The model under review builds one solid part; all positions refer to its coordinate system, in mm. Face numbers are marked on the shaded views. A direction names the side the tool comes from. Coordinates: 2 decimals unless noted, no trailing zeros. Write each loop counter-clockwise with the first axis right and the second up, starting at its lowest first coordinate (ties: lowest second). Pieces come first, ordered by that corner, then holes.
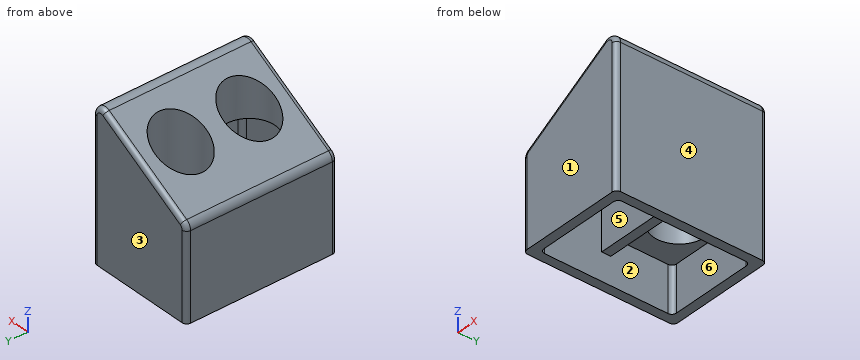
Autodesk Inventor part; units mm, degrees
ref_plane "YZ Plane" through (0, 0, 0) normal (1, 0, 0) x (0, 1, 0)
ref_plane "XZ Plane" through (0, 0, 0) normal (0, 1, 0) x (-1, 0, 0)
ref_plane "XY Plane" through (0, 0, 0) normal (0, 0, 1) x (1, 0, 0)
sketch "Sketch1" plane through (0, 0, 0) normal (0, 1, 0) x (-1, 0, 0)
  line L0 (0, 0) -> (12, 0)
  line L1 (12, 0) -> (12, -10)
  line L2 (12, -10) -> (0, -10)
  line L3 (0, -10) -> (0, 0)
  line L4 (12, 0) -> (0, 6.9282)
  line L5 (12, 0) -> (25.8564, 0) construction
  line L6 (0, 6.9282) -> (0, 0)
  dimension "d0" = 10
  dimension "d1" = 12
  dimension "d2" = 150
extrude "Extrusion1" add sketch "Sketch1" along normal blind 16.5
sketch "Sketch2" plane through (0, 0, -10) normal (0, 0, -1) x (-1, 0, 0)
  circle A0 centre (6, 4.5) radius 2.8
  circle A1 centre (6, 12) radius 2.8
  line L0 (0, 0) -> (0, 16.5)
  line L1 (0, 0) -> (12, 0)
  line L2 (0, 16.5) -> (12, 16.5)
  dimension "d5" = 5.6
  dimension "d6" = 6
  dimension "d7" = 4.5
  dimension "d8" = 4.5
extrude "Extrusion2" cut sketch "Sketch2" against normal through all
fillet "Fillet1" radius 1 2 edges at (0, 8.25, 6.9282) (-12, 8.25, 0)
sketch "Sketch3" plane through (0, 0, -10) normal (0, 0, -1) x (-1, 0, 0)
  circle A0 centre (6, 12) radius 2.8
  circle A1 centre (6, 4.5) radius 2.8
  line L0 (0, 0) -> (12, 0)
  line L1 (12, 0) -> (12, 16.5)
  line L2 (0, 16.5) -> (12, 16.5)
  line L3 (0, 0) -> (0, 16.5)
  line L4 (11, 15.5) -> (11, 1)
  line L5 (11, 1) -> (1, 1)
  line L6 (1, 1) -> (1, 15.5)
  line L7 (1, 15.5) -> (11, 15.5)
  dimension "d12" = 1
extrude "Extrusion3" cut sketch "Sketch3" against normal blind 3 contours L4 L5 L6 L7
fillet "Fillet2" radius 0.5 14 edges at (-0.5, 16.5, 6.0622) (-6.5, 16.5, 3.1754) (-11.866, 16.5, -0.0774) (-12, 16.5, -5.2887) (0, 16.5, -2.4019) (-0.5, 0, 6.0622) (0, 0, -2.4019) (-11.866, 0, -0.0774) (-12, 0, -5.2887) (-6.5, 0, 3.1754) (-1, 15.5, -8.5) (-11, 15.5, -8.5) (-11, 1, -8.5) (-1, 1, -8.5)
sketch "Sketch4" plane through (0, 0, -7) normal (0, 0, -1) x (-1, 0, 0)
  arc A0 (1, 1.5) -> (1.5, 1) centre (1.5, 1.5) ccw
  line L0 (10.5, 1) -> (1.5, 1)
  arc A1 (10.5, 1) -> (11, 1.5) centre (10.5, 1.5) ccw
  line L1 (11, 15) -> (11, 1.5)
  arc A2 (11, 15) -> (10.5, 15.5) centre (10.5, 15) ccw
  line L2 (1.5, 15.5) -> (10.5, 15.5)
  arc A3 (1.5, 15.5) -> (1, 15) centre (1.5, 15) ccw
  line L3 (1, 1.5) -> (1, 15)
  circle A4 centre (6, 4.5) radius 2.8
  circle A5 centre (6, 12) radius 2.8
  line L4 (11, 15) -> (11, 1.5)
  line L5 (11, 7.75) -> (1, 7.75)
  line L6 (1, 1.5) -> (1, 15)
  line L7 (11, 8.75) -> (1, 8.75)
  point P0 (0, 0)
  dimension "d16" = 6.75
  dimension "d17" = 6.75
extrude "Extrusion4" cut sketch "Sketch4" against normal blind 7.5 contours L3 L5 L1 A1 L0 A0
extrude "Extrusion5" cut sketch "Sketch4" against normal blind 2 contours L3 A3 L2 A2 L1 L7
equation "\"d8\" = d7"
properties part number "ProximaCustomCaseFront"
Item 1: Mouldability with a two-part tool opening along Y and no side actions: class the marked faces 3, 4, 5 and 6 as pulls with the +Y half, pulls with the -Y half, needs draft (parallel to the pull), parting line crosses it, or undercut.
Solved:
face 3: pulls with the +Y half
face 4: needs draft
face 5: undercut
face 6: undercut
Item 2: Take a section at B-B, the plane y = 4.5. Write out the cut boundary in (x, z), plus the area to 3 significant figures.
Solved:
outline: (-12, -10) - (-11, -10) - (-11, 0.5) - (-8.8, 0.5) - (-8.8, 1.85) - (-11.5, 0.29) arc R1 ccw to (-12, -0.58) - close; (-3.2, 0.5) - (-1, 0.5) - (-1, -10) - (0, -10) - (0, 5.2) arc R1 ccw to (-1.5, 6.06) - (-3.2, 5.08) - close
area: 39.2 mm2
Item 3: Take a section at A-A, the plane z = -4.5. Write out the cut boundary in (x, y).
Solved:
outline: (-12, 0.5) arc R0.5 ccw to (-11.5, 0) - (-0.5, 0) arc R0.5 ccw to (0, 0.5) - (0, 16) arc R0.5 ccw to (-0.5, 16.5) - (-11.5, 16.5) arc R0.5 ccw to (-12, 16) - close; hole (-11, 1.5) arc R0.5 ccw to (-10.5, 1) - (-1.5, 1) arc R0.5 ccw to (-1, 1.5) - (-1, 7.75) - (-11, 7.75) - close; hole circle Ø5.6 at (-6, 12)
Item 4: Machinability: for the marked faces 1 and 2, which of the approach directions +Z, -Z, +X, -X, +Y, -Y give a long, thin tool a straight path to every point of the face, cutting with its end or side? Answer none if there is none.
Solved:
face 1: +Z, -Z, +X, -X, -Y
face 2: -Z
Item 5: To check wall thickness, follow line 1 along Y through (x, z) = (-6, 2.3); line 2 along Y through (x, z) = (-6, -2.5); line 3 along X through (y, z) = (3.5, -1.5). State the ranges of each line that lie inside material, in increasing order.
Solved:
line 1: y = 0 to 1.7, 7.3 to 9.2, 14.8 to 16.5
line 2: y = 0 to 1, 7.75 to 9.2, 14.8 to 16.5
line 3: x = -12 to -11, -1 to 0
Item 6: Take a section at C-C, the plane z = -7.75. Write out the cut boundary in (x, y).
Solved:
outline: (-12, 0.5) arc R0.5 ccw to (-11.5, 0) - (-0.5, 0) arc R0.5 ccw to (0, 0.5) - (0, 16) arc R0.5 ccw to (-0.5, 16.5) - (-11.5, 16.5) arc R0.5 ccw to (-12, 16) - close; hole (-11, 1.5) arc R0.5 ccw to (-10.5, 1) - (-1.5, 1) arc R0.5 ccw to (-1, 1.5) - (-1, 15) arc R0.5 ccw to (-1.5, 15.5) - (-10.5, 15.5) arc R0.5 ccw to (-11, 15) - close
Item 7: Take a section at D-D, the plane y = 12. Write out the cut boundary in (x, z).
Solved:
outline: (-12, -10) - (-11, -10) - (-11, -5) - (-8.8, -5) - (-8.8, 1.85) - (-11.5, 0.29) arc R1 ccw to (-12, -0.58) - close; (-3.2, -5) - (-1, -5) - (-1, -10) - (0, -10) - (0, 5.2) arc R1 ccw to (-1.5, 6.06) - (-3.2, 5.08) - close
Item 8: For pin 1 (4 mm diameter, centred on x = -3, y = 2.5, fed in from -Z); pin 2 (0.5 mm diameter, centred on x = -7.5, y = 8, fed in from -Z); pin 3 (4 mm diameter, centred on x = -6.5, y = 14, fed in from +Z), all flat-tipped, find the tip position at first contact; note any pin that passes through.
Solved:
pin 1: stops at z = -10
pin 2: stops at z = -7
pin 3: stops at z = 4.31
